For this review, take the finished solid that the model builds, in its own axes (mm). Round coordinates to 2 decimals unless told otherwise and drop trailing zeros. Order: outer loops, then holes, each group sorted by start corner. A loop starts at its lowest first (then second) coordinate and runs counter-clockwise, first axis right, second up. Notation, with made-up numbers: M -14.75,76.5 L -10.75,76.5 A15 ccw -10.75,81.5 Z; hole C -1,42 d9. An arc over 180 degrees is marked long. Use a Markdown table: item, result.
from build123d import *

# Parameters (mm, degrees)
SKETCH1_W           = 455.468181772
SKETCH1_H           = 153.9875
BOSS_EXTRUDE1_DEPTH = 1.5875
SKETCH2_R           = 7.9375
SKETCH2_W           = 6.205681772
SKETCH2_H           = 39.6875
SKETCH2_W_2         = 114.949431772
SKETCH2_H_2         = 48.476800861
CUT_EXTRUDE1_DEPTH  = 1.5875
SKETCH3_R           = 2.667
CUT_EXTRUDE2_DEPTH  = 1.5875


with BuildPart() as part:
    # Sketch1 → Boss-Extrude1 (new body)
    with BuildSketch(Plane(origin=(0, 0, 0), x_dir=(0, 0, -1), z_dir=(1, 0, 0))):
        Rectangle(SKETCH1_W, SKETCH1_H)
    extrude(amount=BOSS_EXTRUDE1_DEPTH)

    # Sketch2 → Cut-Extrude1 (cut)
    with BuildSketch(Plane.ZY):
        with Locations((211.859090932, -54.76875)):
            Circle(SKETCH2_R)
        with Locations((224.63125, 57.15)):
            Rectangle(SKETCH2_W, SKETCH2_H)
        with Locations((86.121875, -52.75534957)):
            Rectangle(SKETCH2_W_2, SKETCH2_H_2)
    extrude(amount=-CUT_EXTRUDE1_DEPTH, mode=Mode.SUBTRACT)

    # Sketch3 → Cut-Extrude2 (cut)
    with BuildSketch(Plane(origin=(1.5875, 0, 0), x_dir=(0, 0, -1), z_dir=(1, 0, 0))):
        with Locations((157.884090886, 55.959375)):
            Circle(SKETCH3_R)
        with Locations((157.884090886, -13.096875)):
            Circle(SKETCH3_R)
        with Locations((30.884090886, -13.096875)):
            Circle(SKETCH3_R)
        with Locations((-45.315909114, -13.096875)):
            Circle(SKETCH3_R)
        with Locations((-172.315909114, -13.096875)):
            Circle(SKETCH3_R)
        with Locations((-172.315909114, 55.959375)):
            Circle(SKETCH3_R)
        with Locations((-45.315909114, 55.959375)):
            Circle(SKETCH3_R)
        with Locations((30.884090886, 55.959375)):
            Circle(SKETCH3_R)
    extrude(amount=-CUT_EXTRUDE2_DEPTH, mode=Mode.SUBTRACT)


solid = part.part
Q1. Clearance check with a flat-ended pin moving along its axis: pin 1 (0.5 mm diameter, centred on x = 1, z = 223.5, fed in from +Y). State where the tip first meets the part, or that it passes through.
Determined:
| item | result |
|---|---|
| pin 1 | stops at y = 37.31 |
Q2. Add section B-B (x = 0.3). Give the number of separate pieces and of enclosed holes in the cut face, then the cut area to 3 significant figures.
Determined:
| item | result |
|---|---|
| separate pieces | 1 |
| enclosed holes | 9 |
| area | 63,900 mm^2 |
Q3. Wall thickness on line 1 along Z through (x, y) = (1, 56); line 2 along Z through (x, y) = (1.5, -61); line 3 along Z through (x, y) = (1.45, 55): over which ranges is each line inside the solid? List them lowest first. Write a range as [from, to].
Determined:
| item | result |
|---|---|
| line 1 | z = [-227.73, -160.55], [-155.22, -33.55], [-28.22, 42.65], [47.98, 169.65], [174.98, 221.53] |
| line 2 | z = [-227.73, 28.65], [143.6, 206.94], [216.78, 227.73] |
| line 3 | z = [-227.73, -160.37], [-155.4, -33.37], [-28.4, 42.83], [47.8, 169.83], [174.8, 221.53] |
Q4. Add section A-A (y = -39). Write out the cut boundary in (x, z).
Determined:
| item | result |
|---|---|
| outline | M 0,-227.73 L 1.59,-227.73 L 1.59,28.65 L 0,28.65 Z; M 0,143.6 L 1.59,143.6 L 1.59,227.73 L 0,227.73 Z |
Q5. Draft analysis for pull direction Y (two halves, no side actions). For faces 1 (the cylindrical face through (0.783, -62.517, 210.138)), 2 (the flat face through (0, 1, 3)), state which applies: pulls with the +Y half, pulls with the -Y half, needs draft (parallel to the pull), parting line crosses it, or undercut.
Determined:
| item | result |
|---|---|
| face 1 | undercut |
| face 2 | needs draft |
Q6. Add section C-C (z = 83.5). Write out the cut boundary in (x, y), then the cut area to 3 significant figures.
Determined:
| item | result |
|---|---|
| outline | M 0,-28.52 L 1.59,-28.52 L 1.59,76.99 L 0,76.99 Z |
| area | 167 mm^2 |
